from build123d import *


# Not quite as in the source:
# - a fillet or chamfer that OpenCascade refuses, or shapes differently, is made with other operations: its cross-section is extruded or revolved along the edge and cut away or added


with BuildPart() as f1:
    # F0 (on Front) → F1 (revolve)
    with BuildSketch(Plane.XZ):
        with BuildLine():
            Line((0, -34), (0, -30))
            Line((0, -30), (-30, -30))
            ThreePointArc((-30, -30), (-39.1968889463, -16.2358830044), (-42.4264068712, 0))
            Line((-42.4264068712, 0), (-50.3107011318, 0))
            Line((-50.3107011318, 0), (-50.3107011318, -4))
            Line((-50.3107011318, -4), (-46.2537701703, -4))
            ThreePointArc((-46.2537701703, -4), (-41.7232145336, -20.361351231), (-31.6134663549, -34))
            Line((-31.6134663549, -34), (0, -34))
        make_face()
    revolve(axis=Axis((0, 0, -15), (0, 0, -1)))

    # F2: fillet of radius 10 on 4 edges, made by hand

    # F2_s1 → F2_t2 (revolve)
    with BuildSketch(Plane.XZ):
        with BuildLine():
            ThreePointArc((-25.5239468456, -30), (-29.9012676169, -28.9910546025), (-33.395292859, -26.1678125731))
            ThreePointArc((-33.395292859, -26.1678125731), (-31.7555066766, -28.135170085), (-30, -30))
            Line((-30, -30), (-25.5239468456, -30))
        make_face()
    revolve(axis=Axis((0, 0, -30), (0, 0, -1)))

    # F2_s3 → F2_t4 (revolve)
    with BuildSketch(Plane.XZ):
        with BuildLine():
            ThreePointArc((-45.2038898575, -10.5839310619), (-47.0388945384, -6.73473945), (-50.3107011318, -4))
            Line((-50.3107011318, -4), (-46.2537701703, -4))
            ThreePointArc((-46.2537701703, -4), (-45.8471692855, -7.310836031), (-45.2038898575, -10.5839310619))
        make_face()
    revolve(axis=Axis((0, 0, -4), (0, 0, -1)))

    # F2_s5 → F2_t6 (revolve, cut)
    with BuildSketch(Plane.XZ):
        with BuildLine():
            ThreePointArc((-50.3107011318, 0), (-44.671276634, -2.6050008536), (-41.6581484398, -8.0373296912))
            ThreePointArc((-41.6581484398, -8.0373296912), (-42.2339055452, -4.0369818424), (-42.4264068712, 0))
            Line((-42.4264068712, 0), (-50.3107011318, 0))
        make_face()
    revolve(axis=Axis((0, 0, 0), (0, 0, -1)), mode=Mode.SUBTRACT)

    # F2_s7 → F2_t8 (revolve, cut)
    with BuildSketch(Plane.XZ):
        with BuildLine():
            ThreePointArc((-34.9248789027, -30.5886267852), (-31.5322424712, -33.1073121131), (-27.4022465784, -34))
            Line((-27.4022465784, -34), (-31.6134663549, -34))
            ThreePointArc((-31.6134663549, -34), (-33.3128685977, -32.3367289744), (-34.9248789027, -30.5886267852))
        make_face()
    revolve(axis=Axis((0, 0, -34), (0, 0, -1)), mode=Mode.SUBTRACT)

    # F3: fillet of radius 5 on 2 edges, made by hand

    # F3_s1 → F3_t2 (revolve, cut)
    with BuildSketch(Plane.XZ):
        with BuildLine():
            ThreePointArc((-48.5206561627, -5.1965315899), (-49.8411412404, -3.478416904), (-50.3107011318, -1.3629707518))
            Line((-50.3107011318, -1.3629707518), (-50.3107011318, -4))
            ThreePointArc((-50.3107011318, -4), (-49.3833812624, -4.5499479973), (-48.5206561627, -5.1965315899))
        make_face()
    revolve(axis=Axis((0, 0, -4), (0, 0, -1)), mode=Mode.SUBTRACT)


solid = f1.part
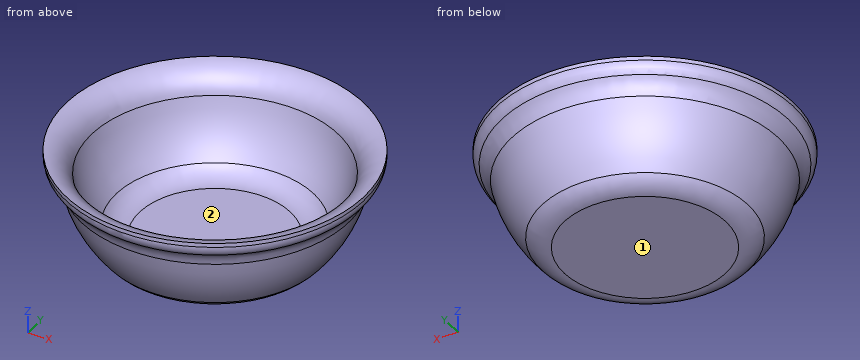
Work out the finished part from the listing and answer in its coordinate system (mm). Face numbers are marked on the shaded views. Give positions to 0.01 mm unless a question says otherwise; leave off trailing zeros. Loops run counter-clockwise (first coordinate to the right, second up) from the corner with the lowest first, then second, coordinate; pieces in that order, holes last. Notation, with made-up numbers: (7.25, 11) - (56.25, 11) arc R38 ccw to (56.25, 49) - close; hole circle Ø8 at (-29, 11). An arc over 180 degrees is marked (long way). Answer in a Markdown table with one row per item.
(1) Section A-A (y = 0) is taken. Give the vertices of the cut face in (x, z).
Results list:
| item | result |
|---|---|
| outline | (-50.31, -1.36) arc R5 ccw to (-48.52, -5.2) arc R10 cw to (-45.2, -10.58) arc R46.43 ccw to (-34.92, -30.59) arc R10 ccw to (-27.4, -34) - (27.4, -34) arc R10 ccw to (34.92, -30.59) arc R46.43 ccw to (45.2, -10.58) arc R10 cw to (48.52, -5.2) arc R5 ccw to (50.31, -1.36) - (50.31, 0) arc R10 ccw to (41.66, -8.04) arc R42.43 cw to (33.4, -26.17) arc R10 cw to (25.52, -30) - (-25.52, -30) arc R10 cw to (-33.4, -26.17) arc R42.43 cw to (-41.66, -8.04) arc R10 ccw to (-50.31, 0) - close |
(2) Section D-D (z = -20) is taken. Give the vertices of the cut face in (x, y).
Results list:
| item | result |
|---|---|
| outline | circle Ø83.8 at (0, 0); hole circle Ø74.83 at (0, 0) |
(3) For a pull along X with two mould halves and no side action, classify the marked faces 1 and 2 as pulls with the +X half, pulls with the -X half, needs draft (parallel to the pull), parting line crosses it, or undercut.
Results list:
| item | result |
|---|---|
| face 1 | needs draft |
| face 2 | undercut |
(4) Consider L1, parallel to Y at x = -21, z = -8.5; L2, parallel to Y at x = 18, z = -24.5; L3, parallel to X at y = 7, z = -18. Determine where each line is inside the solid, lowest interval first. Write a range as [from, to].
Results list:
| item | result |
|---|---|
| L1 | y = [-40.86, -35.87], [35.87, 40.86] |
| L2 | y = [-35.09, -29.59], [29.59, 35.09] |
| L3 | x = [-42.22, -37.78], [37.78, 42.22] |
(5) Flat-ended cylindrical pins translate along their axes: pin 1 Ø2 at (x, y) = (-27, -9.5) entering from +Z; pin 2 Ø4 at (x, z) = (-2, -29.5) entering from +Y; pin 3 Ø3 at (x, z) = (-9, -21.5) entering from -Y. Find the tip coordinate at first contact, or state that the pin passes through.
Results list:
| item | result |
|---|---|
| pin 1 | stops at z = -29.12 |
| pin 2 | stops at y = 37.36 |
| pin 3 | stops at y = -40.99 |
(6) Section C-C (z = -32) is taken. Give the vertices of the cut face in (x, y).
Results list:
| item | result |
|---|---|
| outline | circle Ø66.8 at (0, 0) |
